from build123d import *

# Parameters (mm, degrees)
CROQUIS1_W              = 100
CROQUIS1_H              = 60
SALIENTE_EXTRUIR1_DEPTH = 2
REDONDEO1_R             = 2
SALIENTE_EXTRUIR2_START = 20
SALIENTE_EXTRUIR2_DEPTH = 20


with BuildPart() as part:
    # Croquis1 → Saliente-Extruir1 (new body)
    with BuildSketch(Plane.XY):
        with Locations((50, 30)):
            Rectangle(CROQUIS1_W, CROQUIS1_H)
    extrude(amount=SALIENTE_EXTRUIR1_DEPTH)

    # Redondeo1
    redondeo1_edges = [part.edges().sort_by_distance(p)[0] for p in [
        (0, 60, 1),
        (100, 60, 1),
        (100, 0, 1),
        (0, 0, 1),
    ]]
    fillet(redondeo1_edges, radius=REDONDEO1_R)

    # Croquis2 → Saliente-Extruir2 (add)
    with BuildSketch(Plane.XY.offset(2).offset(SALIENTE_EXTRUIR2_START)):
        with BuildLine():
            Line((70.390057163, 22.374328634), (90.669872981, 57.5))
            ThreePointArc((90.669872981, 57.5), (96.294095226, 59.829629131), (100, 55))
            Line((100, 55), (100, 2))
            ThreePointArc((100, 2), (99.414213562, 0.585786438), (98, 0))
            Line((98, 0), (2, 0))
            ThreePointArc((2, 0), (0.585786438, 0.585786438), (0, 2))
            Line((0, 2), (0, 40))
            Line((0, 40), (10, 40))
            Line((10, 40), (10, 26))
            ThreePointArc((10, 26), (13.504011149, 16.364532168), (22.378965379, 11.230769231))
            ThreePointArc((22.378965379, 11.230769231), (40.620786832, 10.113661458), (58.640126552, 13.165771512))
            ThreePointArc((58.640126552, 13.165771512), (65.406478623, 16.632658786), (70.390057163, 22.374328634))
        make_face()
    extrude(amount=-SALIENTE_EXTRUIR2_DEPTH)


solid = part.part
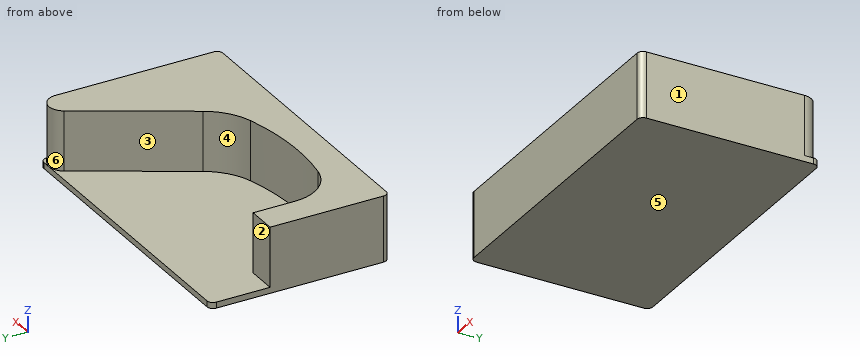
Part model, mm, in its own coordinate system. Face numbers are marked on the shaded views. A direction names the side the tool comes from. Round coordinates to 2 decimals unless told otherwise and drop trailing zeros. Write each loop counter-clockwise with the first axis right and the second up, starting at its lowest first coordinate (ties: lowest second). Pieces come first, ordered by that corner, then holes. Notation, with made-up numbers: M 71.5,34.5 L 80.5,34.5 A32 ccw 80.5,66.5 Z; hole C 11,-23 d4. An arc over 180 degrees is marked long. Return JSON: item names as keys, results as strings. Group by question number.
(1) Saw through at C-C on y = 30. Write the cut outline in (x, z).
(2) Saw through at B-B on z = 3. Write the cut outline in (x, y).
(3) Drill centre lines: probe 1 along Z at (x, y) = (54.5, 46); probe 2 along X at (y, z) = (39, 11.25); probe 3 along X at (y, z) = (20, 4). Where is each one in solid material? Low to high.
(4) Saw through at A-A on x = 6.5. Write the cut outline in (y, z).
(5) Which spindle directions (+Z, -Z, +X, -X, +Y, -Y) get a long thin tool onto all of the face, cutting with end or side? Do the marked faces 1, 2 and 3. Say none if no direction does.
(6) Two-plate mould, pull along X, no slides. Class the marked faces 4, 5 and 6: +X half, -X half, draft (parallel to the pull), parting line (faces both ways), or undercut.
(7) Saw through at D-D on x = 28. Write the cut outline in (y, z), then the cut area to 3 significant figures.
(8) Pin check, flat tips, straight feed: pin 1 Ø6 at (x, y) = (24, 27.5) entering from +Z; pin 2 Ø1 at (x, z) = (43.5, 18.5) entering from +Y; pin 3 Ø3 at (x, z) = (6, 14.5) entering from +Y. Stop position of each tip, or through.
Returned:
{
 "1": {"outline": "M 0,0 L 100,0 L 100,22 L 74.79,22 L 74.79,2 L 10,2 L 10,22 L 0,22 Z"},
 "2": {"outline": "M 0,2 A2 ccw 2,0 L 98,0 A2 ccw 100,2 L 100,55 A5 ccw 90.67,57.5 L 70.39,22.37 A20 cw 58.64,13.17 A80 cw 22.38,11.23 A15 cw 10,26 L 10,40 L 0,40 Z"},
 "3": {"probe 1": "0 to 2", "probe 2": "0 to 10, 79.99 to 100", "probe 3": "0 to 11.25, 68.78 to 100"},
 "4": {"outline": "M 0,0 L 60,0 L 60,2 L 40,2 L 40,22 L 0,22 Z"},
 "5": {"face 1": "+Z, -Z, +X, +Y, -Y", "face 2": "+Z, -X, +Y", "face 3": "+Z, +Y"},
 "6": {"face 4": "undercut", "face 5": "draft", "face 6": "parting line"},
 "7": {"outline": "M 0,0 L 60,0 L 60,2 L 10.44,2 L 10.44,22 L 0,22 Z", "area": "329 mm²"},
 "8": {"pin 1": "z = 2", "pin 2": "y = 10.37", "pin 3": "y = 40"}
}
